Part model, mm, in its own coordinate system. Face numbers are marked on the shaded views. A direction names the side the tool comes from. Coordinates: 2 decimals unless noted, no trailing zeros. Loops run counter-clockwise (first coordinate to the right, second up) from the corner with the lowest first, then second, coordinate; pieces in that order, holes last. Notation, with made-up numbers: M -6,15.25 L 41,15.25 A25 ccw 41,29.25 Z; hole C -27,84 d11. An arc over 180 degrees is marked long. Use a Markdown table: item, result. Add a question column.
1) Band-saw the part on D-D (y = 1.25). State how many separate pieces and enclosed holes the cut face has, plus the area to 3 significant figures.
2) Band-saw the part on B-B (y = -1.5). List the corners of the cut face in (x, z).
3) Wall check: probe 1 along Z at (x, y) = (15, 2.8) (3 decimals); probe 2 along Y at (x, z) = (0, 7.75); probe 3 along Y at (x, z) = (21, 12). Give the ranges that are in metal, low to high. Write a range as from..to.
4) Band-saw the part on A-A (x = 0). List the corners of the cut face in (y, z).
5) Band-saw the part on C-C (z = 3.5). List the corners of the cut face in (x, y).
6) Pull direction Z, two halves, no side cores. Call the marked faces 1, 2 and 3: released by +Z, released by -Z, zero draft, split by the parting line, or undercut.
7) Pin check, flat tips, straight feed: pin 1 Ø3 at (x, z) = (-15, 7.5) entering from +Y; pin 2 Ø5 at (x, z) = (15, 7.5) entering from -Y. Stop position of each tip, or through.
8) Tool access for the marked faces 4, 5 and 6: list every direction of +Z, -Z, +X, -X, +Y, -Y with a clear straight run to the whole face (end or side of a thin tool).
from build123d import *

# Parameters (mm, degrees)
F0_R        = 2.5
F1_DEPTH    = 15
F3_D        = 3.25
F4_T1_DEPTH = 45
F4_T3_DEPTH = 45.0017535366


# Not quite as in the source:
# - a fillet or chamfer that OpenCascade refuses, or shapes differently, is made with other operations: its cross-section is extruded or revolved along the edge and cut away or added


with BuildPart() as f1:
    # F0 (on Top) → F1 (new body)
    with BuildSketch(Plane.XY):
        with BuildLine():
            Line((6, 0), (23.4290786547, 0))
            Line((23.4290786547, 0), (23.5615114343, 5))
            Line((23.5615114343, 5), (-21.4384885657, 5))
            Line((-21.4384885657, 5), (-21.4384885657, 0))
            Line((-21.4384885657, 0), (-6, 0))
            ThreePointArc((-6, 0), (0, -6), (6, 0))
        make_face()
        Circle(F0_R, mode=Mode.SUBTRACT)
    extrude(amount=F1_DEPTH)

    # F3 (through all)
    with Locations(Plane.XZ):
        with Locations((-15, 7.5), (15, 7.5)):
            Hole(F3_D / 2)

    # F4: fillet of radius 8 on 4 edges, made by hand

    # F4_s2 → F4_t1 (cut)
    with BuildSketch(Plane.XZ.offset(-25)):
        with BuildLine():
            ThreePointArc((-13.4384885657, 15), (-19.0953428152, 12.6568542495), (-21.4384885657, 7))
            Line((-21.4384885657, 7), (-21.4384885657, 15))
            Line((-21.4384885657, 15), (-13.4384885657, 15))
        make_face()
        with BuildLine():
            ThreePointArc((-13.4384885657, 0), (-19.0953428152, 2.3431457505), (-21.4384885657, 8))
            Line((-21.4384885657, 8), (-21.4384885657, 0))
            Line((-21.4384885657, 0), (-13.4384885657, 0))
        make_face()
    extrude(amount=F4_T1_DEPTH, mode=Mode.SUBTRACT)

    # F4_s4 → F4_t3 (cut)
    with BuildSketch(Plane(origin=(-0.5131205452, -19.3728677482, 0), x_dir=(0, 0, 1), z_dir=(0.0264772702, 0.9996494156, 0))):
        with BuildLine():
            ThreePointArc((15, 15.4208647858), (12.6568542495, 21.0777190353), (7, 23.4208647858))
            Line((7, 23.4208647858), (15, 23.4208647858))
            Line((15, 23.4208647858), (15, 15.4208647858))
        make_face()
        with BuildLine():
            ThreePointArc((0, 15.4208647858), (2.3431457505, 21.0777190353), (8, 23.4208647858))
            Line((8, 23.4208647858), (0, 23.4208647858))
            Line((0, 23.4208647858), (0, 15.4208647858))
        make_face()
    extrude(amount=F4_T3_DEPTH, mode=Mode.SUBTRACT)


solid = f1.part
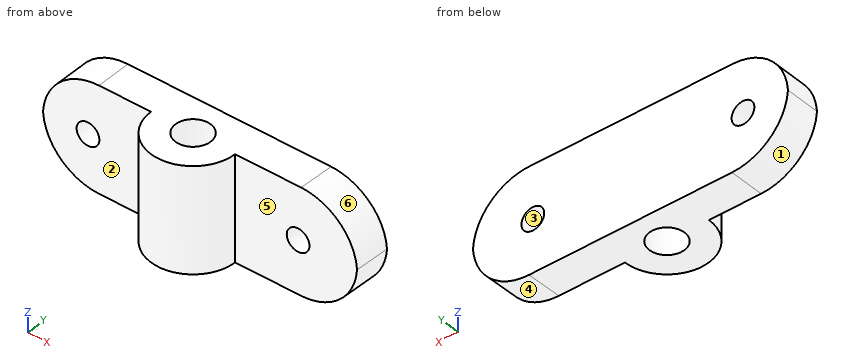
Entries:
| question | item | result |
|---|---|---|
| 1 | separate pieces | 2 |
| 1 | enclosed holes | 2 |
| 1 | area | 537 mm2 |
| 2 | outline | M -5.81,0 L -2,0 L -2,15 L -5.81,15 Z; M 2,0 L 5.81,0 L 5.81,15 L 2,15 Z |
| 3 | probe 1 | 0..5.875, 9.125..15 |
| 3 | probe 2 | -6..-2.5, 2.5..5 |
| 3 | probe 3 | 0..5 |
| 4 | outline | M -6,0 L -2.5,0 L -2.5,15 L -6,15 Z; M 2.5,0 L 5,0 L 5,15 L 2.5,15 Z |
| 5 | outline | M -20.05,0 L -6,0 A6 ccw 6,0 L 22.04,0 L 22.18,5 L -20.05,5 Z; hole C 0,0 d5 |
| 6 | face 1 | released by -Z |
| 6 | face 2 | zero draft |
| 6 | face 3 | undercut |
| 7 | pin 1 | through |
| 7 | pin 2 | y = 0 |
| 8 | face 4 | -Z, +X, -Y |
| 8 | face 5 | +Z, -Z, +X, -Y |
| 8 | face 6 | +Z, +X, -Y |
